Geometry: see drawing. Coordinates: mm, zero at the bounding-box minimum. A direction names the side the tool comes from. Round coordinates to 2 decimals unless told otherwise and drop trailing zeros. Write each loop counter-clockwise with the first axis right and the second up, starting at its lowest first coordinate (ties: lowest second). Pieces come first, ordered by that corner, then holes.
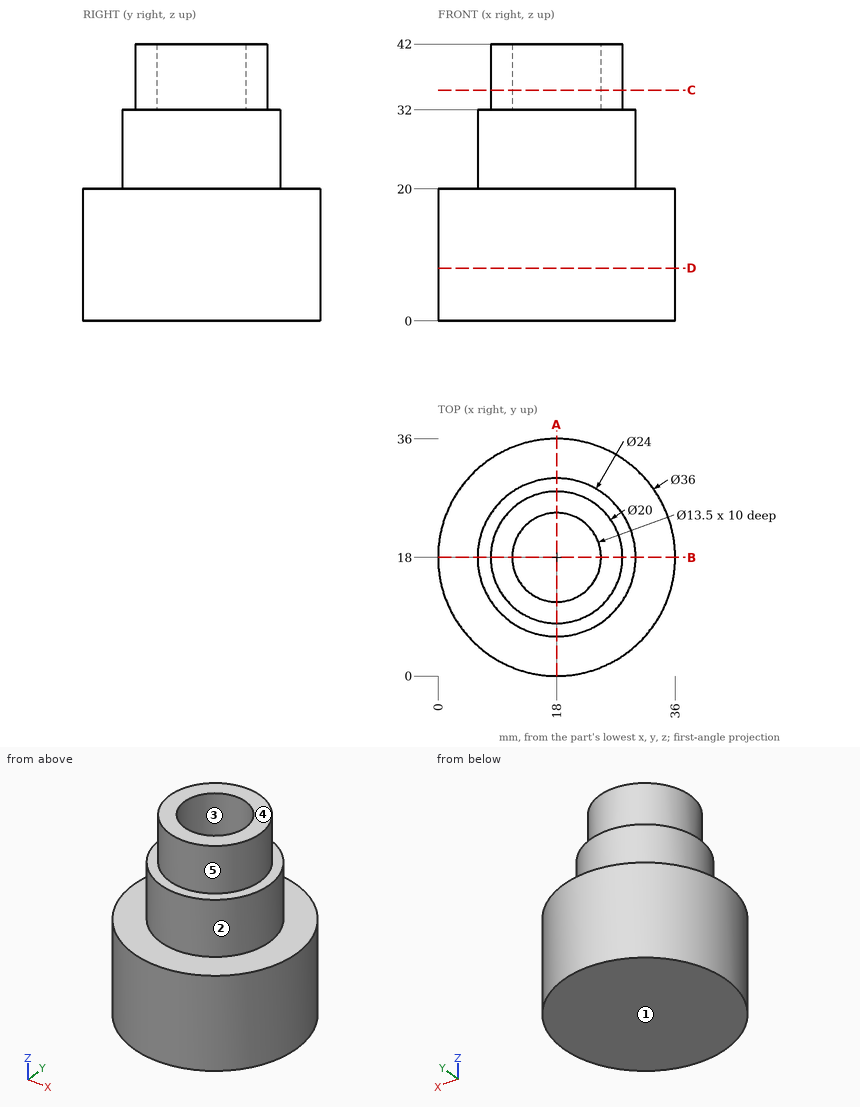
1) Pull-direction query (X, two-part tool) for the marked faces 1, 2 and 3; classes: released by +X, released by -X, zero draft, split by the parting line, or undercut.
Taken from the geometry:
face 1: zero draft
face 2: split by the parting line
face 3: undercut
2) Section query D-D on z = 8. Return the cut outline in (x, y).
Taken from the geometry:
outline: circle Ø36 at (18, 18)
3) Contact query for flat-ended pins moving along their axis: P1, Ø6, axis at y = 28.5, z = 27, coming from the +X side; P2, Ø1, axis at y = 4.5, z = 12.5, coming from the +X side; P3, Ø10, axis at x = 22.5, z = 34.5, coming from the +Y side; P4, Ø2, axis at y = 5, z = 33.5, coming from the +X side. Output: stop coordinate, or through.
Taken from the geometry:
P1: stops at x = 27.37
P2: stops at x = 30.45
P3: stops at y = 30
P4: passes through
4) Section query A-A on x = 18. Return the cut outline in (y, z), then the cut area to 3 significant figures.
Taken from the geometry:
outline: (0, 0) - (36, 0) - (36, 20) - (30, 20) - (30, 32) - (28, 32) - (28, 42) - (24.75, 42) - (24.75, 32) - (11.25, 32) - (11.25, 42) - (8, 42) - (8, 32) - (6, 32) - (6, 20) - (0, 20) - close
area: 1,070 mm2
5) Section query C-C on z = 35. Return the cut outline in (x, y), then the cut area to 3 significant figures.
Taken from the geometry:
outline: circle Ø20 at (18, 18); hole circle Ø13.5 at (18, 18)
area: 171 mm2
6) Reachability of the marked faces 4 and 5 from +Z, -Z, +X, -X, +Y, -Y: full face, straight path, thin tool, end or side. Return the list, or none.
Taken from the geometry:
face 4: +Z, +X, -X, +Y, -Y
face 5: +Z
7) Material intervals for line 1 (Y direction, x = 18, z = 35.5); line 2 (Z direction, x = 5.5, y = 10); line 3 (Z direction, x = 8, y = 16.5), sorted ascending.
Taken from the geometry:
line 1: y = 8 to 11.25, 24.75 to 28
line 2: z = 0 to 20
line 3: z = 0 to 32
